Input: part model. Units: mm. Frame: model coordinates. Face numbers are marked on the shaded views. A direction names the side the tool comes from. Coordinates: 2 decimals unless noted, no trailing zeros. Write each loop counter-clockwise with the first axis right and the second up, starting at its lowest first coordinate (ties: lowest second). Pieces come first, ordered by that corner, then holes. Notation, with made-up numbers: (4, 40.5) -> (58, 40.5) arc R11 cw to (58, 44.5) -> close; hole circle Ø7 at (13, -5). An arc over 180 degrees is marked (long way). Use one line per item in the form item = value. Start each with the question number.
(1) Cut plane D-D on x = -22. Return the cut outline in (y, z).
(2) Set-up query: the marked faces 1, 2 and 3. Return all of +Z, -Z, +X, -X, +Y, -Y with unobstructed straight access to the full face (end or side cutting, diameter ignored); none if empty.
(3) Pull-direction query (Z, two-part tool) for the marked faces 4, 5 and 6; classes: released by +Z, released by -Z, zero draft, split by the parting line, or undercut.
(4) Cut plane B-B on z = 0. Return the cut outline in (x, y).
(5) Cut plane A-A on x = 0. Return the cut outline in (y, z), plus the area to 3 significant figures.
(6) Cut plane C-C on y = 3.25. State how many separate pieces and enclosed holes the cut face has, plus the area to 3 significant figures.
(7) Ray query, line 1 along X through (y, z) = (3.25, 1); line 2 along Z through (x, y) = (0, 8.4); line 3 along X through (y, z) = (8.5, 0). Return the intervals inside material, ascending.
(8) First-contact query: pin 1 (1.5 mm diameter, centred on y = 7.5, z = -12.5, fed in from -X); pin 2 (15.5 mm diameter, centred on x = -4.5, z = 1.5, fed in from +Y); pin 3 (1.5 mm diameter, centred on x = -18, z = -15, fed in from -Y). Flat tips, straight axial feed; report the tip coordinate or a pass-through.
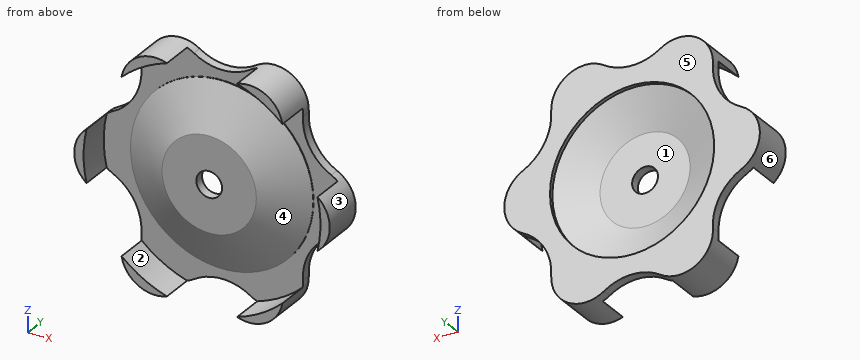
```python
from build123d import *

# Parameters (mm, degrees)
SKETCH_7_OUTSIDE_W  = 72.02
SKETCH_7_OUTSIDE_H  = 72.02
CUT_EXTRUDE_3_DEPTH = 11


with BuildPart() as part:
    # 草图4 → 旋转-薄壁1 (revolve)
    with BuildSketch(Plane.XY):
        Polygon((2.75, 4.5), (9.608214533, 4.5), (17.5, 8.18), (17.5, 9), (27.25, 9), (27.25, 0), (25.25, 0), (25.25, 7), (19.5, 7), (19.5, 6.905859478), (10.051603858, 2.5), (2.75, 2.5), align=None)
    revolve(axis=Axis((0, 0, 0), (0, 1, 0)))

    # 草图7 outside → 切除-拉伸3 (cut)
    with BuildSketch(Plane(origin=(0, 0, 0), x_dir=(1, 0, 0), z_dir=(0, 1, 0))):
        Rectangle(SKETCH_7_OUTSIDE_W, SKETCH_7_OUTSIDE_H)
        with BuildLine():
            ThreePointArc((23.265907271, -6.472738964), (27.25, 0), (23.265907271, 6.472738964))
            ThreePointArc((23.265907271, 6.472738964), (18.694797481, 10.793446358), (17.23851001, 16.912497256))
            ThreePointArc((17.23851001, 16.912497256), (13.625, 23.599192253), (6.02739726, 23.385236221))
            ThreePointArc((6.02739726, 23.385236221), (0, 21.586892716), (-6.02739726, 23.385236221))
            ThreePointArc((-6.02739726, 23.385236221), (-13.625, 23.599192253), (-17.23851001, 16.912497256))
            ThreePointArc((-17.23851001, 16.912497256), (-18.694797481, 10.793446358), (-23.265907271, 6.472738964))
            ThreePointArc((-23.265907271, 6.472738964), (-27.25, 0), (-23.265907271, -6.472738964))
            ThreePointArc((-23.265907271, -6.472738964), (-18.694797481, -10.793446358), (-17.23851001, -16.912497256))
            ThreePointArc((-17.23851001, -16.912497256), (-13.625, -23.599192253), (-6.02739726, -23.385236221))
            ThreePointArc((-6.02739726, -23.385236221), (0, -21.586892716), (6.02739726, -23.385236221))
            ThreePointArc((6.02739726, -23.385236221), (13.625, -23.599192253), (17.23851001, -16.912497256))
            ThreePointArc((17.23851001, -16.912497256), (18.694797481, -10.793446358), (23.265907271, -6.472738964))
        make_face(mode=Mode.SUBTRACT)
    extrude(amount=CUT_EXTRUDE_3_DEPTH, mode=Mode.SUBTRACT)


solid = part.part
```
Values:
q1.outline = (7, -7.22) -> (9, -7.22) -> (9, 7.22) -> (7, 7.22) -> close
q2.face_1 = +Y
q2.face_2 = -Y
q2.face_3 = +X, +Y, -Y
q3.face_4 = undercut
q3.face_5 = zero draft
q3.face_6 = split by the parting line
q4.outline = (-27.25, 0) -> (-25.25, 0) -> (-25.25, 7) -> (-19.5, 7) -> (-19.5, 6.91) -> (-10.05, 2.5) -> (-2.75, 2.5) -> (-2.75, 4.5) -> (-9.61, 4.5) -> (-17.5, 8.18) -> (-17.5, 9) -> (-27.25, 9) -> close; (2.75, 2.5) -> (10.05, 2.5) -> (19.5, 6.91) -> (19.5, 7) -> (25.25, 7) -> (25.25, 0) -> (27.25, 0) -> (27.25, 9) -> (17.5, 9) -> (17.5, 8.18) -> (9.61, 4.5) -> (2.75, 4.5) -> close
q5.outline = (2.5, -10.05) -> (6.91, -19.5) -> (7, -19.5) -> (7, -21.59) -> (9, -21.59) -> (9, -17.5) -> (8.18, -17.5) -> (4.5, -9.61) -> (4.5, -2.75) -> (2.5, -2.75) -> close; (2.5, 2.75) -> (4.5, 2.75) -> (4.5, 9.61) -> (8.18, 17.5) -> (9, 17.5) -> (9, 21.59) -> (7, 21.59) -> (7, 19.5) -> (6.91, 19.5) -> (2.5, 10.05) -> close
q5.area = 80.8 mm2
q6.separate_pieces = 7
q6.enclosed_holes = 1
q6.area = 498 mm2
q7.line_1 = -27.18 to -25.23, -11.62 to -2.56, 2.56 to 11.62, 25.23 to 27.18
q7.line_2 = -21.59 to -17.5, 17.5 to 21.59
q7.line_3 = -27.25 to -17.5, 17.5 to 27.25
q8.pin_1 = -18.2
q8.pin_2 = 5.85
q8.pin_3 = 7
